The model under review builds one solid part; all positions refer to its coordinate system, in mm. Coordinates: 2 decimals unless noted, no trailing zeros. Loops run counter-clockwise (first coordinate to the right, second up) from the corner with the lowest first, then second, coordinate; pieces in that order, holes last. Notation, with made-up numbers: M 68.25,38.5 L 104.25,38.5 A15 ccw 104.25,46.5 Z; hole C 4,80.25 d4. An arc over 180 degrees is marked long. Write item = value, one per line. Start each with the question number.
Q1. Clearance check with flat-ended pins moving along their axes: pin 1 Ø1 at (x, y) = (-63.5, 22.5) entering from +Z; pin 2 Ø4 at (y, z) = (17, 66.5) entering from +X. State where each tip first meets the part, or that it passes through.
Q2. We need section B-B on x = -172. Give the boundary of the cut face in (y, z) (3 decimals), and give its area (3 significant figures).
Q3. We need section A-A on y = 17.5. Give the boundary of the cut face in (x, z).
Q4. Mouldability with a two-part tool opening along Z and no side actions: class faces 1 (the face through (-611, 20, 62)), 2 (the face through (-202.04, 28.952, 128.671)), 3 (the face through (-196.46, 28.95, -3.63)), 4 (the face through (-537, 24.5, 71)) as released by +Z, released by -Z, zero draft, split by the parting line, or undercut.
Q5. Wall thickness on probe 1 along Z at (x, y) = (-431, 14); probe 2 along Z at (x, y) = (-274, 26.75); probe 3 along Y at (x, z) = (-94, 125.5): over which ranges is each line inside the solid? List them lowest first.
Autodesk Inventor part; units mm, degrees
ref_plane "Work Plane1" through (-461.6, 0, 0) normal (1, 0, 0) x (0, 1, 0)
ref_plane "XZ Plane" through (0, 0, 0) normal (0, 1, 0) x (-1, 0, 0)
ref_plane "XY Plane" through (0, 0, 0) normal (0, 0, 1) x (1, 0, 0)
sketch "Sketch4" plane through (0, 0, 0) normal (1, 0, 0) x (0, 1, 0)
  circle A0 centre (20.1532, 0.0226) radius 9.525
  circle A1 centre (20.1532, 0.0226) radius 9.525
  dimension "d10" = 19.05
  dimension "d21" = 19.05
sketch "Sketch5" plane through (0, 0, 0) normal (0, 1, 0) x (-1, 0, 0)
  line L0 (0, 9.5476) -> (0, -9.5024)
  line L1 (398.5, 0.0226) -> (0, 0.0226)
  arc A0 (398.5, 0.0226) -> (398.5, 125.0226) centre (398.5, 62.5226) ccw
  line L2 (398.5, 62.5226) -> (398.5, 125.0226) construction
  line L3 (398.5, 62.5226) -> (398.5, 0.0226) construction
  line L4 (398.5, 125.0226) -> (0, 125.0226)
  line L5 (461, 62.5226) -> (611, 62.5226)
  dimension "d14" = 398.5
  dimension "d15" = 125
  dimension "d18" = 150
sweep "Sweep4" add profiles "Sketch4" path "Sketch5" path curves L1 A0 L4
ref_plane "Work Plane1" through (-461.6, 0, 0) normal (1, 0, 0) x (0, 1, 0)
sketch "Sketch8" plane through (-461.6, 0, 0) normal (1, 0, 0) x (0, 1, 0)
  circle A0 centre (20.1532, 125.0226) radius 9.525
  circle A1 centre (20.1532, 0.0226) radius 9.525
  line L0 (20.1532, 125.0226) -> (20.1532, 0.0226)
  circle A2 centre (20.1532, 62.5226) radius 9.525
  dimension "d24" = 19.05
sweep "Sweep5" add profiles "Sketch8" path "Sketch5" path curves L5 contours A2 L0 | L0 A2
properties part number "Y_ancla"
Returned:
q1.pin_1 = 134.37
q1.pin_2 = -451.35
q2.outline = C 20.153,0.023 d19.05; C 20.153,125.023 d19.05
q2.area = 570 mm^2
q3.outline = M -611,53.37 L -469.56,53.37 A71.65 ccw -398.5,-9.13 L 0,-9.13 L 0,9.17 L -398.5,9.17 A53.35 cw -398.5,115.87 L 0,115.87 L 0,134.17 L -398.5,134.17 A71.65 ccw -469.56,71.67 L -611,71.67 Z
q4.face_1 = zero draft
q4.face_2 = undercut
q4.face_3 = undercut
q4.face_4 = split by the parting line
q5.probe_1 = 0.78 to 17.87, 107.18 to 124.26
q5.probe_2 = -6.85 to 6.89, 118.15 to 131.89
q5.probe_3 = 10.64 to 29.67
